The listing builds one solid part. Answer for the finished solid, in the listing's coordinates (mm). A direction names the side the tool comes from. Round coordinates to 2 decimals unless told otherwise and drop trailing zeros. Order: outer loops, then holes, each group sorted by start corner. A loop starts at its lowest first (then second) coordinate and runs counter-clockwise, first axis right, second up. Notation, with made-up numbers: (84.25, -18) -> (92.25, -18) arc R13 ccw to (92.25, -6) -> close; hole circle Ø6 at (36, 65). An arc over 180 degrees is marked (long way). Return JSON: item names as keys, results as strings. Group by question number.
(1) The part is cut by section A-A (z = 6.25). Determine the outline of the cut face in (x, y).
(2) The part is cut by section B-B (y = 5.75). Determine the outline of the cut face in (x, z).
(3) Consider line 1 (Z direction, x = 6, y = 4); line 2 (Z direction, x = 29.5, y = 0.75); line 3 (Y direction, x = 23, z = -2.75). Determine where each line is inside the solid, lowest interval first. Write a range as [from, to].
(4) Determine the mould class of faces 1 (the face through (15, 0, 0)), 2 (the face through (15, 2, 10)), 3 (the face through (15, 3, -6.6)) for opening direction Z: +Z half, -Z half, draft (parallel to the pull), parting line (faces both ways), or undercut.
(5) Which of the six approach directions +Z, -Z, +X, -X, +Y, -Y give full straight-line access (tool end or side, diameter ignored) to faces 4 (the face through (15, 0, 9)), 5 (the face through (15.21, 4.699, 2.685)), 6 (the face through (15.21, 4.715, 6.299))?
(6) Each of these flat-tipped pins is pushed along its axis until it touches: pin 1 (4 mm diameter, centred on x = 27, y = 7, fed in from -Z); pin 2 (10 mm diameter, centred on x = 9.5, z = 5, fed in from +Y); pin 3 (1.5 mm diameter, centred on x = 15, z = 4.5, fed in from +Y); pin 4 (2.5 mm diameter, centred on x = 17.5, z = -5, fed in from -Y). Where does it stop, or does it pass through?
Autodesk Inventor part; units mm, degrees
ref_plane "YZ Plane" through (0, 0, 0) normal (1, 0, 0) x (0, 1, 0)
ref_plane "XZ Plane" through (0, 0, 0) normal (0, 1, 0) x (-1, 0, 0)
ref_plane "XY Plane" through (0, 0, 0) normal (0, 0, 1) x (1, 0, 0)
sketch "Szkic1" plane through (0, 0, 0) normal (1, 0, 0) x (0, 1, 0)
  line L0 (0, 0) -> (10, 0) construction
  line L1 (0, 0) -> (0, -3.6)
  line L2 (0, -3.6) -> (2, -3.6)
  line L3 (2, -3.6) -> (2, -2.4)
  line L4 (2, -2.4) -> (5, -2.4)
  line L5 (5, -2.4) -> (5, -6.6)
  line L6 (5, -6.6) -> (0, -6.6)
  arc A0 (3.5826, -10) -> (10, 0) centre (-1, 0) ccw
  line L7 (0, 0) -> (0, 3.6)
  line L8 (0, 3.6) -> (2, 3.6)
  line L9 (2, 3.6) -> (2, 2.4)
  line L10 (2, 2.4) -> (5, 2.4)
  line L11 (5, 2.4) -> (5, 6.6)
  line L12 (5, 6.6) -> (0, 6.6)
  arc A1 (10, 0) -> (3.5826, 10) centre (-1, 0) ccw
  line L13 (3.5826, -10) -> (0, -10)
  line L14 (0, -10) -> (0, -6.6)
  line L15 (0, 6.6) -> (0, 10)
  line L16 (0, 10) -> (3.5826, 10)
  dimension "d10" = 3.6
  dimension "d13" = 3
  dimension "d14" = 11
  dimension "d19" = 5
  dimension "d22" = 10
  dimension "d28" = 10
  dimension "d29" = 4.2
  dimension "d32" = 3
  dimension "d34" = 2
extrude "Wyciągnięcie proste1" add sketch "Szkic1" along normal blind 30
fillet "Zaokrąglenie2" radius 1 12 edges at (15, 5, -2.4) (15, 5, -6.6) (15, 2, -3.6) (15, 0, -3.6) (15, 0, 3.6) (15, 2, 3.6) (15, 2, 2.4) (15, 5, 2.4) (15, 5, 6.6) (15, 0, 6.6) (15, 0, -6.6) (15, 2, -2.4)
properties part number "wciskacz_v2" material "PLA"
Answer below:
{
 "1": {"outline": "(0, 4.76) -> (30, 4.76) -> (30, 8.05) -> (0, 8.05) -> close"},
 "2": {"outline": "(0, -8.69) -> (30, -8.69) -> (30, 8.69) -> (0, 8.69) -> close"},
 "3": {"line 1": "z = [-9.8, -6.6], [-2.4, 2.4], [6.6, 9.8]", "line 2": "z = [-10, -6.63], [-3.57, 3.57], [6.63, 10]", "line 3": "y = [0.01, 2.24], [4.76, 9.65]"},
 "4": {"face 1": "draft", "face 2": "+Z half", "face 3": "undercut"},
 "5": {"face 4": "+Z, -Z, +X, -X, -Y", "face 5": "+X, -X", "face 6": "+X, -X, -Y"},
 "6": {"pin 1": "stops at z = -9.22", "pin 2": "stops at y = 10", "pin 3": "stops at y = 9.34", "pin 4": "stops at y = 4.76"}
}
